Here's how the part is built. I have some questions about the finished solid (model axes, mm). A direction names the side the tool comes from. Round coordinates to 2 decimals unless told otherwise and drop trailing zeros. Loops run counter-clockwise (first coordinate to the right, second up) from the corner with the lowest first, then second, coordinate; pieces in that order, holes last. Notation, with made-up numbers: (85.5, 74.25) - (132.5, 74.25) arc R21 cw to (132.5, 97.25) - close; hole circle Ø6 at (-25, 26). An arc over 180 degrees is marked (long way). Return JSON: item names as keys, results as strings. Group by question number.
```python
from build123d import *

# Parameters (mm, degrees)
SKETCH1_R           = 10
BOSS_EXTRUDE1_DEPTH = 4
SKETCH2_R           = 5
BOSS_EXTRUDE2_DEPTH = 7
SKETCH3_R           = 1.5
BOSS_EXTRUDE3_DEPTH = 7
FILLET4_R           = 7.4
FILLET15_R          = 4.2
FILLET16_R          = 3


with BuildPart() as part:
    # Sketch1 → Boss-Extrude1 (new body)
    with BuildSketch(Plane.XY):
        Circle(SKETCH1_R)
    extrude(amount=BOSS_EXTRUDE1_DEPTH)

    # Sketch2 → Boss-Extrude2 (add)
    with BuildSketch(Plane.XY.offset(4)):
        Circle(SKETCH2_R)
    extrude(amount=BOSS_EXTRUDE2_DEPTH)

    # Sketch3 → Boss-Extrude3 (add)
    with BuildSketch(Plane.XY.offset(11)):
        Circle(SKETCH3_R)
    extrude(amount=BOSS_EXTRUDE3_DEPTH)

    # Fillet4
    # the kernel refuses this fillet: 7.4 mm, written as the material it adds along each edge
    with BuildSketch(Plane(origin=(0, 0, 4), x_dir=(1, 0, 0), z_dir=(0, -1, 0))) as fillet4_piece_1:
        with BuildLine():
            CenterArc((12.4, 7), FILLET4_R, 180, 71.075355584)
            Line((5, 7), (4.852, 7))
            Line((4.852, 7), (4.852, 0))
            Line((4.852, 0), (5, -0.148))
            ThreePointArc((5, -0.148), (7.5, -0.148), (9.952, -0.14))
            Line((9.952, -0.14), (10, 0))
        make_face()
    revolve(axis=Axis((0, 0, 4), (0, 0, 1)))

    # Fillet15
    # the kernel refuses this fillet: 4.2 mm, written as the material it takes off along each edge
    with BuildSketch(Plane(origin=(0, 0, 0), x_dir=(1, 0, 0), z_dir=(0, -1, 0))) as fillet15_piece_1:
        with BuildLine():
            CenterArc((5.804764607, 4.2), FILLET15_R, 270, 87.270597363)
            Line((5.804764607, 0), (5.804764607, -0.084))
            Line((5.804764607, -0.084), (10, -0.084))
            Line((10, -0.084), (10.084, 0))
            ThreePointArc((10.084, 0), (10.084, 2), (10.083904708, 3.996))
            Line((10.083904708, 3.996), (10, 4))
        make_face()
    revolve(axis=Axis((0, 0, 0), (0, 0, 1)), mode=Mode.SUBTRACT)

    # Fillet16
    fillet16_edges = [part.edges().sort_by_distance(p)[0] for p in [
        (-10, 0, 4),
    ]]
    fillet(fillet16_edges, radius=FILLET16_R)


solid = part.part
```
Q1. Please list where these lines run through material, in increasing order: line 1 (Z direction, x = -1.5, y = 2.25); line 2 (Y direction, x = 0, z = 16.5); line 3 (Y direction, x = -2, z = 7.75).
Q2. Will these pins go through, and if not, where does the flat tip stop? pin 1 Ø3 at (x, z) = (-4, 14.5) entering from +Y; pin 2 Ø6 at (x, z) = (2.5, 13.5) entering from -Y.
Q3. Imagine slicing it at A-A, the plane z = 12.5. List the corners of the cut face in (x, y) for me, and give its area (3 significant figures).
Q4. Imagine slicing it at B-B, the plane z = 9.75. List the corners of the cut face in (x, y) for me, and give its area (3 significant figures).
Q5. For faces 1 (the cylindrical face through (-1.5, 0.07, 14.45)), 2 (the flat face through (0, 0, 18)), which set-ups out of +Z, -Z, +X, -X, +Y, -Y let a thin tool reach every point of the face, with its end or its side?
Output values:
{
 "1": {"line 1": "z = 0 to 11", "line 2": "y = -1.5 to 1.5", "line 3": "y = -5.39 to 5.39"},
 "2": {"pin 1": "passes through", "pin 2": "stops at y = -4.93"},
 "3": {"outline": "circle Ø3 at (0, 0)", "area": "7.07 mm^2"},
 "4": {"outline": "circle Ø10.21 at (0, 0)", "area": "81.9 mm^2"},
 "5": {"face 1": "+Z", "face 2": "+Z, +X, -X, +Y, -Y"}
}
